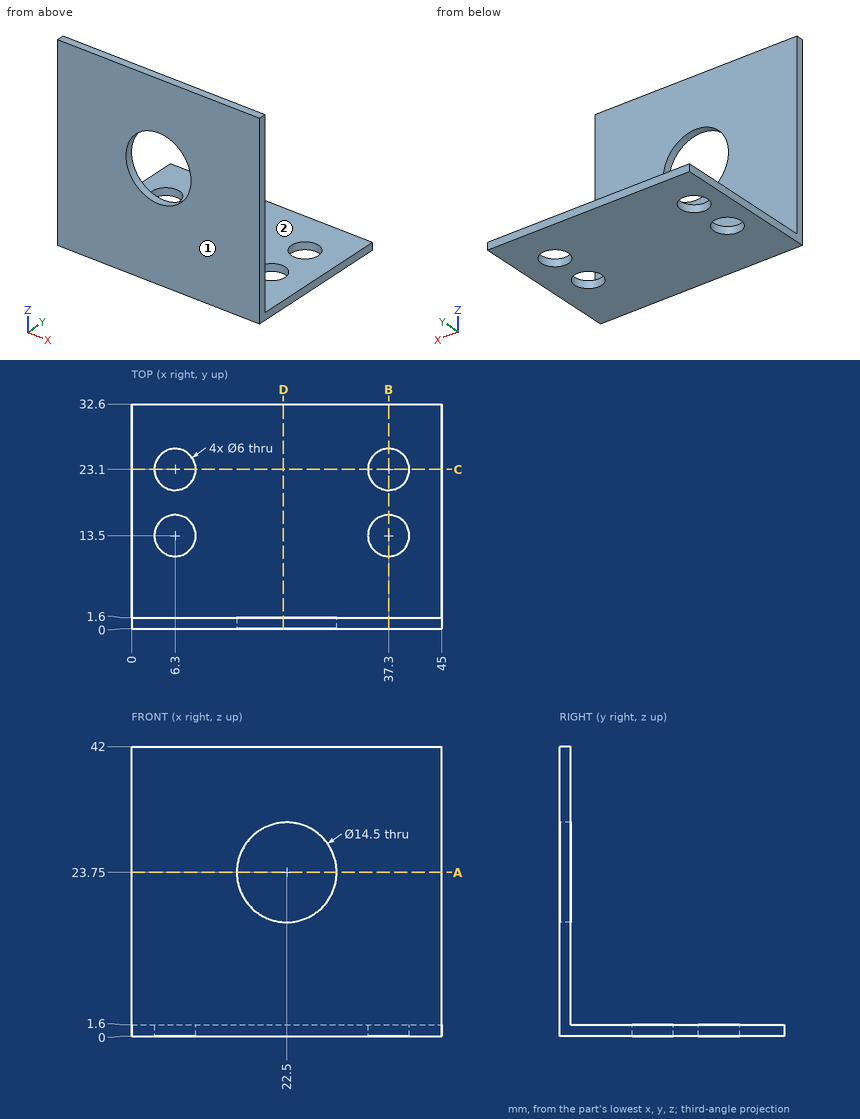
Drawing for the job (mm, zero at the part's lowest x, y, z). A direction names the side the tool comes from. Round coordinates to 2 decimals unless told otherwise and drop trailing zeros. Loops run counter-clockwise (first coordinate to the right, second up) from the corner with the lowest first, then second, coordinate; pieces in that order, holes last. Notation, with made-up numbers: (72.5, 81.5) -> (101.5, 81.5) arc R17 ccw to (101.5, 110.5) -> close; hole circle Ø10 at (88.25, 73). An arc over 180 degrees is marked (long way). Use one line per item in the form item = value. Start each with the question number.
Item 1: Band-saw the part on C-C (y = 23.1). List the corners of the cut face in (x, z), plus the area to 3 significant figures.
Item 2: Drop flat-ended pins along their axis: pin 1 Ø20 at (x, z) = (20, 19.5) entering from +Y; pin 2 Ø7 at (x, y) = (6.3, 23.1) entering from +Z. Give the stop position or say it passes through.
Item 3: Tool access for the marked faces 1 and 2: list every direction of +Z, -Z, +X, -X, +Y, -Y with a clear straight run to the whole face (end or side of a thin tool).
Item 4: Drill centre lines: line 1 along Y through (x, z) = (6.3, 0.9); line 2 along X through (y, z) = (23.1, 0.5); line 3 along Z through (x, y) = (22.5, 0.5). Where is each one in solid material? Low to high.
Item 5: Band-saw the part on B-B (x = 37.3). List the corners of the cut face in (y, z), plus the area to 3 significant figures.
Item 6: Band-saw the part on A-A (z = 23.75). List the corners of the cut face in (x, y).
Item 7: Band-saw the part on D-D (x = 22). List the corners of the cut face in (y, z), plus the area to 3 significant figures.
Data:
q1.outline = (0, 0) -> (3.3, 0) -> (3.3, 1.6) -> (0, 1.6) -> close; (9.3, 0) -> (34.3, 0) -> (34.3, 1.6) -> (9.3, 1.6) -> close; (40.3, 0) -> (45, 0) -> (45, 1.6) -> (40.3, 1.6) -> close
q1.area = 52.8 mm^2
q2.pin_1 = 1.6
q2.pin_2 = 1.6
q3.face_1 = +Z, -Z, +X, -X, -Y
q3.face_2 = +Z, +X, -X, +Y
q4.line_1 = 0 to 10.5, 16.5 to 20.1, 26.1 to 32.6
q4.line_2 = 0 to 3.3, 9.3 to 34.3, 40.3 to 45
q4.line_3 = 0 to 16.5, 31 to 42
q5.outline = (0, 0) -> (10.5, 0) -> (10.5, 1.6) -> (1.6, 1.6) -> (1.6, 42) -> (0, 42) -> close; (16.5, 0) -> (20.1, 0) -> (20.1, 1.6) -> (16.5, 1.6) -> close; (26.1, 0) -> (32.6, 0) -> (32.6, 1.6) -> (26.1, 1.6) -> close
q5.area = 97.6 mm^2
q6.outline = (0, 0) -> (15.25, 0) -> (15.25, 1.6) -> (0, 1.6) -> close; (29.75, 0) -> (45, 0) -> (45, 1.6) -> (29.75, 1.6) -> close
q7.outline = (0, 0) -> (32.6, 0) -> (32.6, 1.6) -> (1.6, 1.6) -> (1.6, 16.52) -> (0, 16.52) -> close; (0, 30.98) -> (1.6, 30.98) -> (1.6, 42) -> (0, 42) -> close
q7.area = 93.7 mm^2
